Check sheet for the drawn part. Datum: minimum x, y, z corner. Units: mm. A direction names the side the tool comes from. Round coordinates to 2 decimals unless told otherwise and drop trailing zeros. Write each loop counter-clockwise with the first axis right and the second up, starting at its lowest first coordinate (ties: lowest second). Pieces come first, ordered by that corner, then holes.
Item 1: Material ranges on line 1 (X direction, y = 1, z = 12); line 2 (Y direction, x = 20, z = 24.3); line 3 (Y direction, x = 32.5, z = 13.25), recorded low to high.
Item 2: Go/stop test with flat-tipped pins: pin 1 Ø8 at (x, y) = (10, 7.5) entering from -Z; pin 2 Ø11.5 at (x, z) = (21, 17) entering from +Y. Record where each tip stops, or that it passes through.
Item 3: Tool access check on the marked faces 1 and 2. Record the directions out of +Z, -Z, +X, -X, +Y, -Y that give a thin tool (end or side, any length) a straight path to the whole face; none if there is none.
Item 4: Cross-section at D-D on x = 20. Enter the section's corners in (y, z), plus the area to 3 significant figures.
Item 5: Cross-section at C-C on z = 12. Enter the section's corners in (x, y).
Item 6: Cross-section at B-B on x = 5. Enter the section's corners in (y, z), plus the area to 3 significant figures.
Item 7: Cross-section at A-A on y = 13. Enter the section's corners in (x, z).
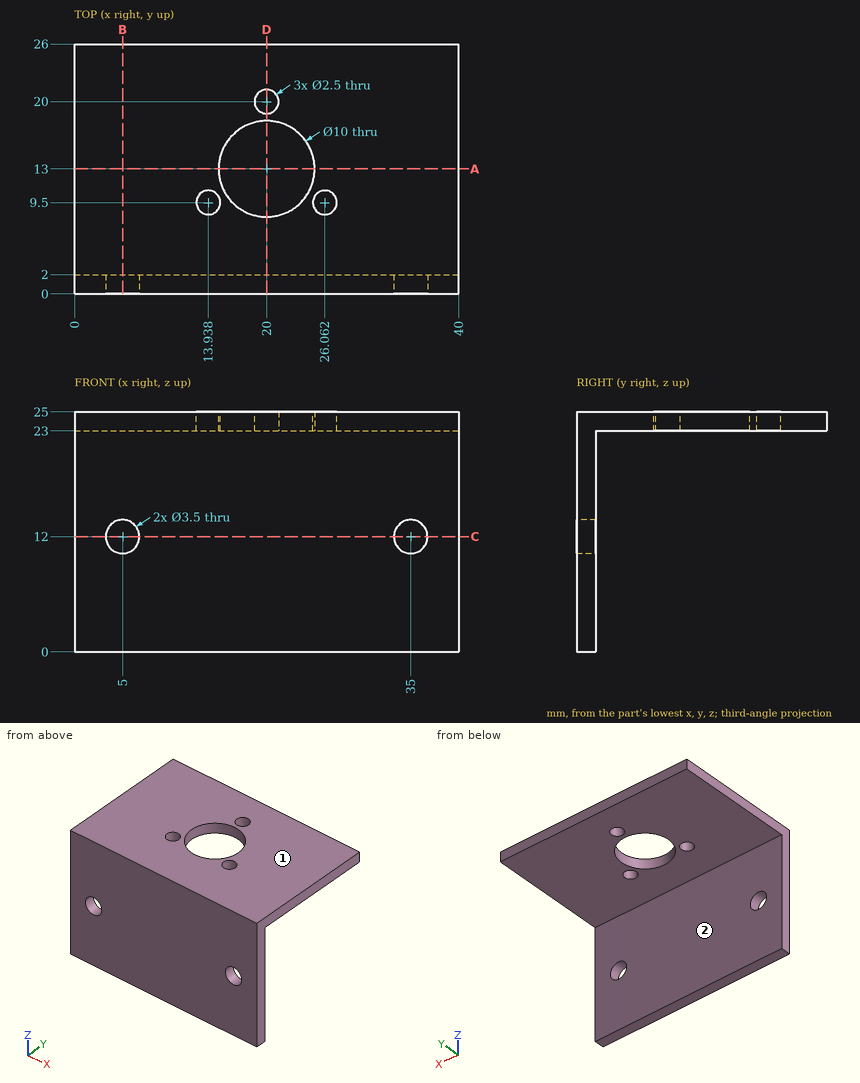
Response values:
1. line 1: x = 0 to 3.25, 6.75 to 33.25, 36.75 to 40
1. line 2: y = 0 to 8, 18 to 18.75, 21.25 to 26
1. line 3: y = 0 to 2
2. pin 1: stops at z = 23
2. pin 2: stops at y = 2
3. face 1: +Z, +X, -X, +Y, -Y
3. face 2: -Z, +X, -X, +Y
4. outline: (0, 0) - (2, 0) - (2, 23) - (8, 23) - (8, 25) - (0, 25) - close; (18, 23) - (18.75, 23) - (18.75, 25) - (18, 25) - close; (21.25, 23) - (26, 23) - (26, 25) - (21.25, 25) - close
4. area: 73.0 mm2
5. outline: (0, 0) - (3.25, 0) - (3.25, 2) - (0, 2) - close; (6.75, 0) - (33.25, 0) - (33.25, 2) - (6.75, 2) - close; (36.75, 0) - (40, 0) - (40, 2) - (36.75, 2) - close
6. outline: (0, 0) - (2, 0) - (2, 10.25) - (0, 10.25) - close; (0, 13.75) - (2, 13.75) - (2, 23) - (26, 23) - (26, 25) - (0, 25) - close
6. area: 91.0 mm2
7. outline: (0, 23) - (15, 23) - (15, 25) - (0, 25) - close; (25, 23) - (40, 23) - (40, 25) - (25, 25) - close
